For this review, use the dimensioned drawing (mm, ordinates from the lowest corner) and the shaded views. Give positions to 0.01 mm unless a question says otherwise; leave off trailing zeros. Write each loop counter-clockwise with the first axis right and the second up, starting at its lowest first coordinate (ties: lowest second). Pieces come first, ordered by that corner, then holes. Notation, with made-up numbers: M 82,77.5 L 129,77.5 A24 ccw 129,115.5 Z; hole C 47,77 d5. An arc over 180 degrees is marked long. Answer in a Markdown table with one row per item.
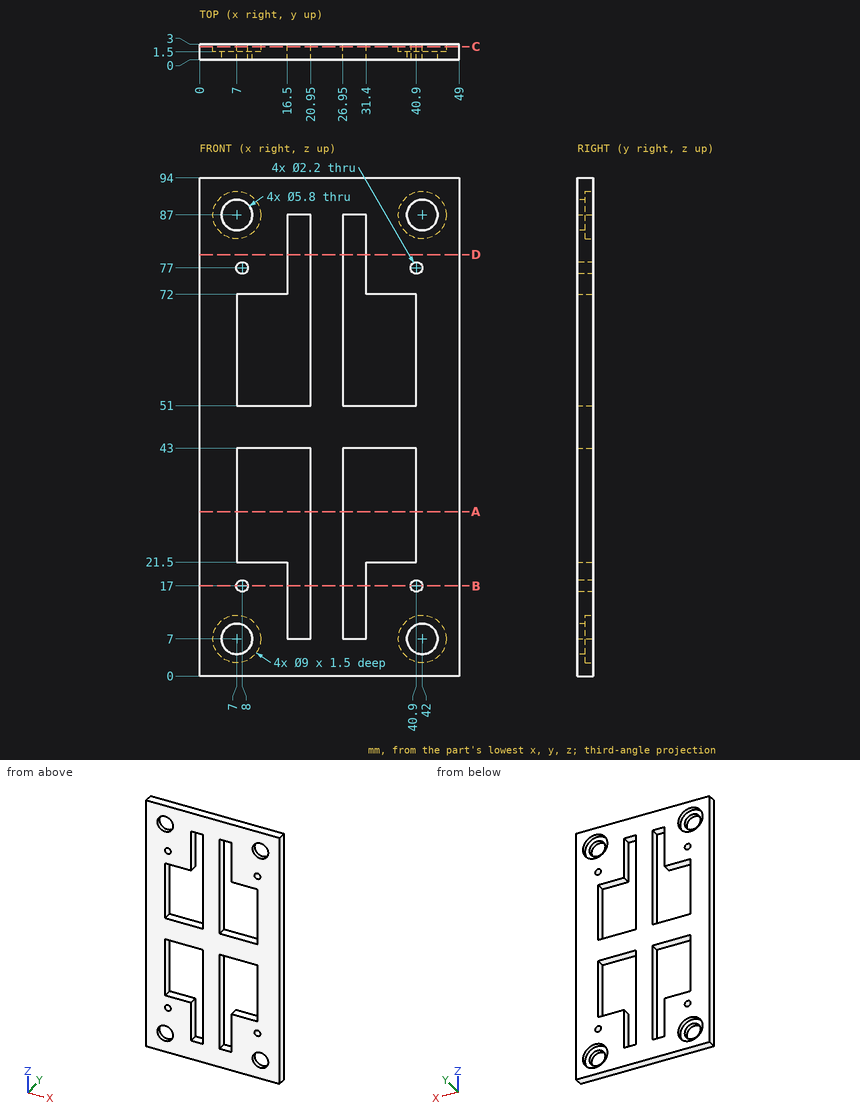
1) Add section D-D (z = 79.5). Write out the cut boundary in (x, y), and give its area (3 significant figures).
Geometry says:
| item | result |
|---|---|
| outline | M 0,0 L 16.5,0 L 16.5,3 L 0,3 Z; M 20.95,0 L 26.95,0 L 26.95,3 L 20.95,3 Z; M 31.4,0 L 49,0 L 49,3 L 31.4,3 Z |
| area | 120 mm^2 |
2) Add section B-B (z = 17). Write out the cut boundary in (x, y), and give its area (3 significant figures).
Geometry says:
| item | result |
|---|---|
| outline | M 0,0 L 6.9,0 L 6.9,3 L 0,3 Z; M 9.1,0 L 16.5,0 L 16.5,3 L 9.1,3 Z; M 20.95,0 L 26.95,0 L 26.95,3 L 20.95,3 Z; M 31.4,0 L 39.8,0 L 39.8,3 L 31.4,3 Z; M 42,0 L 49,0 L 49,3 L 42,3 Z |
| area | 107 mm^2 |
3) Add section A-A (z = 31). Write out the cut boundary in (x, y), and give its area (3 significant figures).
Geometry says:
| item | result |
|---|---|
| outline | M 0,0 L 7,0 L 7,3 L 0,3 Z; M 20.95,0 L 26.95,0 L 26.95,3 L 20.95,3 Z; M 40.9,0 L 49,0 L 49,3 L 40.9,3 Z |
| area | 63.3 mm^2 |
4) Add section C-C (y = 2.5). Count the separate pieces of the cut face and the enclosed holes in it, and give its area (3 significant figures).
Geometry says:
| item | result |
|---|---|
| separate pieces | 1 |
| enclosed holes | 12 |
| area | 2,890 mm^2 |
5) To check wall thickness, follow probe 1 along X at (y, z) = (1.3, 33); probe 2 along Z at (x, y) = (14, 0.6); probe 3 along X at (y, z) = (0.9, 17). State the ranges of each line that lie inside material, in increasing order. Write a range as [from, to].
Geometry says:
| item | result |
|---|---|
| probe 1 | [0, 7], [20.95, 26.95], [40.9, 49] |
| probe 2 | [0, 21.5], [43, 51], [72, 94] |
| probe 3 | [0, 6.9], [9.1, 16.5], [20.95, 26.95], [31.4, 39.8], [42, 49] |
6) Insertion check: P1, Ø6.5, axis at x = 7, z = 87, coming from the +Y side. The pin has a flat end and moves straight along its axis. Give the tip position at first contact, or say it passes through.
Geometry says:
| item | result |
|---|---|
| P1 | y = 1.5 |
